Autodesk Inventor part; units mm, degrees
ref_plane "YZ Plane" through (0, 0, 0) normal (1, 0, 0) x (0, 1, 0)
ref_plane "XZ Plane" through (0, 0, 0) normal (0, 1, 0) x (-1, 0, 0)
ref_plane "XY Plane" through (0, 0, 0) normal (0, 0, 1) x (1, 0, 0)
sketch "Sketch1" plane through (0, 0, 0) normal (0, 1, 0) x (-1, 0, 0)
  line L0 (-50, 50) -> (-50, -50)
  line L1 (-50, -50) -> (50, -50)
  line L2 (50, -50) -> (50, 50)
  line L3 (50, 50) -> (-50, 50)
  line L4 (-50, 50) -> (50, -50) construction
  line L5 (-50, -50) -> (50, 50) construction
  point P0 (0, 0)
  dimension "d0" = 100
  dimension "d1" = 100
extrude "Extrusion1" add sketch "Sketch1" along normal blind 110
sketch "Sketch2" plane through (0, 110, 0) normal (0, 1, 0) x (1, 0, 0)
  line L0 (40, -40) -> (40, 40)
  line L1 (40, 40) -> (-40, 40)
  line L2 (-40, 40) -> (-40, -40)
  line L3 (-40, -40) -> (40, -40)
  line L4 (40, -40) -> (-40, 40) construction
  line L5 (40, 40) -> (-40, -40) construction
  point P0 (0, 0)
  dimension "d4" = 80
  dimension "d5" = 80
extrude "Extrusion2" cut sketch "Sketch2" against normal blind 110
sketch "Sketch3" plane through (50, 0, 50) normal (1, 0, 0) x (0, 0, -1)
  line L0 (50, 0) -> (50, 110) construction
  line L1 (90, 110) -> (10, 110) construction
  line L2 (0, 0) -> (0, 110) construction
  line L3 (0, 110) -> (100, 0) construction
  line L4 (100, 0) -> (100, 110) construction
  line L5 (100, 0) -> (100, 110) construction
  line L6 (0, 0) -> (100, 0) construction
  line L7 (100, 110) -> (0, 0) construction
  line L8 (10, 10) -> (90, 10)
  line L9 (90, 10) -> (90, 100)
  line L10 (90, 100) -> (10, 100)
  line L11 (10, 100) -> (10, 10)
  line L12 (10, 10) -> (90, 100) construction
  line L13 (90, 10) -> (10, 100) construction
  point P0 (50, 55)
  dimension "d8" = 90
extrude "Extrusion3" cut sketch "Sketch3" against normal through all
sketch "Sketch4" plane through (-50, 0, 50) normal (0, 0, 1) x (1, 0, 0)
  line L0 (0, 0) -> (100, 0)
  line L1 (100, 0) -> (100, 110)
  line L2 (0, 110) -> (100, 110)
  line L3 (0, 0) -> (0, 110)
  line L4 (10, 10) -> (10, 0)
  line L5 (90, 0) -> (10, 0)
  line L6 (90, 10) -> (90, 0)
  line L7 (100, 10) -> (90, 10)
  line L8 (100, 100) -> (100, 10)
  line L9 (100, 100) -> (90, 100)
  line L10 (90, 110) -> (90, 100)
  line L11 (10, 110) -> (90, 110)
  line L12 (10, 110) -> (10, 100)
  line L13 (10, 100) -> (0, 100)
  line L14 (0, 10) -> (0, 100)
  line L15 (10, 10) -> (0, 10)
  line L16 (0, 110) -> (100, 0) construction
  line L17 (0, 110) -> (100, 110) construction
  line L18 (100, 110) -> (0, 0) construction
  line L19 (10, 10) -> (90, 10)
  line L20 (90, 10) -> (90, 100)
  line L21 (90, 100) -> (10, 100)
  line L22 (10, 100) -> (10, 10)
  line L23 (10, 10) -> (90, 100) construction
  line L24 (90, 10) -> (10, 100) construction
  point P0 (50, 0)
  point P1 (50, 55)
extrude "Extrusion4" cut sketch "Sketch4" against normal through all contours L22 L21 L20 L19
sketch "Sketch5" plane through (0, 0, 0) normal (0, -1, 0) x (1, 0, 0)
  line L0 (-40, 40) -> (-50, 40)
  line L1 (-50, 40) -> (-45, 40)
  line L2 (-45, 40) -> (-45, 45)
  line L3 (-50, 50) -> (50, 50)
  line L4 (-45, 45) -> (-40, 45)
  line L5 (-40, 50) -> (-40, 40)
  line L6 (-40, 45) -> (-40, 50)
  line L7 (-50, 40) -> (-50, 50)
  line L8 (-50, 50) -> (-40, 50)
  line L9 (-40, 50) -> (0, 50)
  line L10 (-40, 45) -> (0, 45)
  line L11 (0, 56.6181) -> (0, 31.8895) construction
  line L12 (45, 40) -> (50, 40)
  line L13 (45, 40) -> (45, 45)
  line L14 (50, 50) -> (-50, 50)
  line L15 (45, 45) -> (40, 45)
  line L16 (40, 50) -> (40, 45)
  line L17 (50, 40) -> (50, 50)
  line L18 (40, 45) -> (0, 45)
  point P0 (0, 0)
  point P1 (40, 40)
  dimension "d13" = 5
  dimension "d14" = 5
  dimension "d15" = 5
extrude "Extrusion5" add sketch "Sketch5" along normal blind 10 contours L0 L7 L3 L5 L4 L2 | L16 L3 L17 L12 L13 L15
sketch "Sketch6" plane through (0, 0, 0) normal (0, -1, 0) x (1, 0, 0)
  line L0 (-40, 45) -> (-40, 50)
  line L1 (-40, 45) -> (40, 45)
  line L2 (40, 45) -> (40, 50)
  line L3 (40, 45) -> (40, 50)
  line L4 (40, 50) -> (-40, 50)
  line L5 (-40, 50) -> (-40, 45)
  point P0 (0, 0)
extrude "Extrusion6" add sketch "Sketch6" along normal blind 5
sketch "Sketch7" plane through (0, 0, 0) normal (0, -1, 0) x (1, 0, 0)
  line L0 (50, -50) -> (-50, -50)
  line L1 (50, -50) -> (50, -40)
  line L2 (50, 40) -> (50, -50)
  line L3 (50, -40) -> (45, -40)
  line L4 (50, -40) -> (40, -40)
  line L5 (45, -40) -> (50, -40)
  line L6 (45, -40) -> (45, -45)
  line L7 (45, -45) -> (40, -45)
  line L8 (40, -45) -> (40, -50)
  line L9 (40, -45) -> (-40, -45)
  line L10 (-40, -40) -> (-40, -50)
  line L11 (-40, -50) -> (-40, -45)
  line L12 (40, -40) -> (40, -50)
  line L13 (-40, -50) -> (40, -50)
  line L14 (40, -50) -> (-40, -50)
  line L15 (-40, -45) -> (-45, -45)
  line L16 (-45, -45) -> (-45, -40)
  line L17 (-45, -40) -> (-50, -40)
  line L18 (-40, -50) -> (-50, -50)
  line L19 (-50, -50) -> (-50, 50)
  line L20 (-50, -40) -> (-50, -50)
  point P0 (0, 0)
  dimension "d20" = 10
  dimension "d21" = 5
  dimension "d22" = 5
  dimension "d23" = 5
extrude "Extrusion7" add sketch "Sketch7" along normal blind 10 contours L0 L8 L7 L6 L3 L1 | L0 L19 L17 L16 L15 L10
extrude "Extrusion8" add sketch "Sketch7" along normal blind 5 contours L0 L10 L9 L8
sketch "Sketch8" plane through (-40, 110, -40) normal (0, 0, 1) x (1, 0, 0)
  line L0 (80, -10) -> (0, -10)
  line L1 (0, -10) -> (0, -5)
  line L2 (0, -5) -> (80, -5)
  line L3 (80, -5) -> (80, -10)
  point P0 (40, -110)
  dimension "d28" = 5
extrude "Extrusion9" add sketch "Sketch8" along normal blind 2
sketch "Sketch9" plane through (40, 110, -40) normal (-1, 0, 0) x (0, 0, 1)
  line L0 (80, -10) -> (0, -10)
  line L1 (0, -10) -> (0, -5)
  line L2 (0, -5) -> (80, -5)
  line L3 (80, -100) -> (80, -10)
  line L4 (80, -5) -> (80, -10)
  point P0 (40, -110)
  dimension "d31" = 5
extrude "Extrusion10" add sketch "Sketch9" along normal blind 2
sketch "Sketch10" plane through (40, 110, 40) normal (0, 0, -1) x (-1, 0, 0)
  line L0 (80, -10) -> (0, -10)
  line L1 (0, -10) -> (0, -5)
  line L2 (0, -5) -> (80, -5)
  line L3 (80, -5) -> (80, -10)
  point P0 (40, -110)
  dimension "d34" = 5
  dimension "d35" = 80
extrude "Extrusion11" add sketch "Sketch10" along normal blind 2
sketch "Sketch11" plane through (-40, 110, 40) normal (1, 0, 0) x (0, 0, -1)
  line L0 (80, -10) -> (0, -10)
  line L1 (0, -10) -> (0, -5)
  line L2 (0, -5) -> (80, -5)
  line L3 (80, -5) -> (80, -10)
  point P0 (40, -110)
  dimension "d38" = 5
  dimension "d39" = 80
extrude "Extrusion12" add sketch "Sketch11" along normal blind 2
properties part number "Lifting Main Frame"
Source: CAD feature listing. Evaluate the final solid. Frame: model axes, mm. A direction names the side the tool comes from. Coordinates: 2 decimals unless noted, no trailing zeros. Loops run counter-clockwise (first coordinate to the right, second up) from the corner with the lowest first, then second, coordinate; pieces in that order, holes last. Notation, with made-up numbers: M 78,-23 L 96,-23 A29 ccw 96,-2 Z; hole C 77,53 d5. An arc over 180 degrees is marked long. Answer in a Markdown table with one row per item.
Q1. Section B-B on z = 41.5. Return the cut outline in (x, y).
Answers below:
| item | result |
|---|---|
| outline | M -50,-10 L -45,-10 L -45,0 L 45,0 L 45,-10 L 50,-10 L 50,110 L -50,110 Z; hole M -40,10 L 40,10 L 40,100 L -40,100 Z |
Q2. Section A-A on y = 90. Return the cut outline in (x, z), plus the area to 3 significant figures.
Answers below:
| item | result |
|---|---|
| outline | M -50,-50 L -40,-50 L -40,-40 L -50,-40 Z; M -50,40 L -40,40 L -40,50 L -50,50 Z; M 40,-50 L 50,-50 L 50,-40 L 40,-40 Z; M 40,40 L 50,40 L 50,50 L 40,50 Z |
| area | 400 mm^2 |
Q3. Ray query, probe 1 along X at (y, z) = (102, -23); probe 2 along Y at (x, z) = (44.5, 32); probe 3 along X at (y, z) = (3, 37.5). Return the intervals inside material, ascending. Write a range as from..to.
Answers below:
| item | result |
|---|---|
| probe 1 | x = -50..-38, 38..50 |
| probe 2 | y = 0..10, 100..110 |
| probe 3 | x = -50..-40, 40..50 |
Q4. Set-up query: faces 1 (the flat face through (40, 108, 1)), 2 (the flat face through (-1, -5, -47)), 3 (the flat face through (-40, 56, -45)), 4 (the flat face through (38, 103, -1)), 5 (the flat face through (1, 5, 40)). Return all of +Z, -Z, +X, -X, +Y, -Y with unobstructed straight access to the full face (end or side cutting, diameter ignored); none if empty.
Answers below:
| item | result |
|---|---|
| face 1 | +Y |
| face 2 | +Z, -Z, -Y |
| face 3 | +Z, -Z |
| face 4 | +Y, -Y |
| face 5 | -Y |
Q5. Section C-C on y = 4. Return the cut outline in (x, z), plus the area to 3 significant figures.
Answers below:
| item | result |
|---|---|
| outline | M -50,-50 L 50,-50 L 50,50 L -50,50 Z; hole M -40,-40 L 40,-40 L 40,40 L -40,40 Z |
| area | 3,600 mm^2 |
Q6. First-contact query: pin 1 (10 mm diameter, centred on x = 38, y = 42, fed in from +Z); pin 2 (4 mm diameter, centred on x = -37.5, y = 88.5, fed in from +Z); pin 3 (4 mm diameter, centred on x = -18, z = -47, fed in from -Y). Flat tips, straight axial feed; report the tip coordinate or a pass-through.
Answers below:
| item | result |
|---|---|
| pin 1 | stops at z = 50 |
| pin 2 | passes through |
| pin 3 | stops at y = -5 |
Q7. Section D-D on x = 25.5. Return the cut outline in (y, z).
Answers below:
| item | result |
|---|---|
| outline | M -5,-50 L 10,-50 L 10,-40 L 0,-40 L 0,-45 L -5,-45 Z; M -5,45 L 0,45 L 0,40 L 10,40 L 10,50 L -5,50 Z; M 100,-50 L 110,-50 L 110,-40 L 105,-40 L 105,-38 L 100,-38 Z; M 100,38 L 105,38 L 105,40 L 110,40 L 110,50 L 100,50 Z |
Q8. Draft query along X for faces 6 (the flat face through (-50, 9, -1)), 7 (the flat face through (-47, -5, 40)), 8 (the flat face through (-45, -5, 42)). Return one class per face: pulls with the +X half, pulls with the -X half, needs draft (parallel to the pull), parting line crosses it, or undercut.
Answers below:
| item | result |
|---|---|
| face 6 | pulls with the -X half |
| face 7 | needs draft |
| face 8 | undercut |
